Build history of the part. All positions in model axes, mm. Round coordinates to 2 decimals unless told otherwise and drop trailing zeros. Write each loop counter-clockwise with the first axis right and the second up, starting at its lowest first coordinate (ties: lowest second). Pieces come first, ordered by that corner, then holes. Notation, with made-up numbers: M 66,-18 L 111,-18 A26 cw 111,20 Z; hole C -32,16.25 d2. An arc over 180 degrees is marked long. Write item = value, one per line.
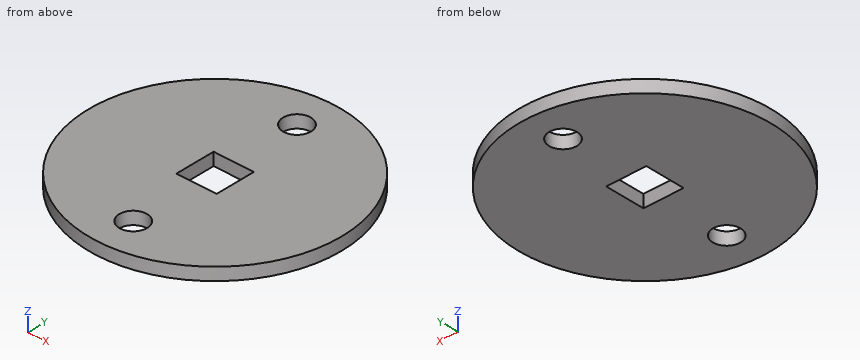
from build123d import *

# Parameters (mm, degrees)
SKETCH1_R          = 10
SKETCH1_R_2        = 1.1
BASE_FLANGE1_DEPTH = 1
CUT_EXTRUDE1_DEPTH = 10


# Sheet-metal steps are written as plain solids
with BuildPart() as part:
    # Sketch1 → Base-Flange1 (new body)
    with BuildSketch(Plane.XY):
        Circle(SKETCH1_R)
        with Locations((0, 7)):
            Circle(SKETCH1_R_2, mode=Mode.SUBTRACT)
        with Locations((0, -7)):
            Circle(SKETCH1_R_2, mode=Mode.SUBTRACT)
    extrude(amount=-BASE_FLANGE1_DEPTH)

    # Sketch6 → Cut-Extrude1 (cut)
    with BuildSketch(Plane.XY):
        Polygon((1.59, 0), (1.59, 1.59), (-1.59, 1.59), (-1.59, -1.59), (1.59, -1.59), align=None)
    extrude(amount=-CUT_EXTRUDE1_DEPTH, mode=Mode.SUBTRACT)


solid = part.part
1. Band-saw the part on A-A (y = 0). List the corners of the cut face in (x, z).
Responses:
outline = M -10,-1 L -1.59,-1 L -1.59,0 L -10,0 Z; M 1.59,-1 L 10,-1 L 10,0 L 1.59,0 Z
2. Band-saw the part on B-B (z = -0.8). List the corners of the cut face in (x, y), plus the area to 3 significant figures.
Responses:
outline = C 0,0 d20; hole M -1.59,-1.59 L 1.59,-1.59 L 1.59,1.59 L -1.59,1.59 Z; hole C 0,-7 d2.2; hole C 0,7 d2.2
area = 296 mm²
3. Band-saw the part on D-D (x = 5.75). List the corners of the cut face in (y, z), plus the area to 3 significant figures.
Responses:
outline = M -8.18,-1 L 8.18,-1 L 8.18,0 L -8.18,0 Z
area = 16.4 mm²
4. Band-saw the part on C-C (y = -7). List the corners of the cut face in (x, z).
Responses:
outline = M -7.14,-1 L -1.1,-1 L -1.1,0 L -7.14,0 Z; M 1.1,-1 L 7.14,-1 L 7.14,0 L 1.1,0 Z
5. Flat gauge pins, fed straight in: pin 1 (6 mm diameter, centred on x = 2.5, y = 2, fed in from +Z); pin 2 (0.5 mm diameter, centred on y = -0.5, z = -0.5, fed in from -X); pin 3 (0.5 mm diameter, centred on x = 0.5, z = -0.5, fed in from -Y). Where does each tip first touch, or does it go through?
Responses:
pin_1 = 0
pin_2 = -10
pin_3 = -10
6. Probe probe 1 along Y at (x, z) = (0, -0.6); probe 2 along Y at (x, z) = (-0.5, -0.75); probe 3 along X at (y, z) = (7.5, -0.7). List the from-to ranges inside material, lowest first.
Responses:
probe_1 = -10 to -8.1, -5.9 to -1.59, 1.59 to 5.9, 8.1 to 10
probe_2 = -9.99 to -7.98, -6.02 to -1.59, 1.59 to 6.02, 7.98 to 9.99
probe_3 = -6.61 to -0.98, 0.98 to 6.61
